Part model, mm, in its own coordinate system. A direction names the side the tool comes from. Coordinates: 2 decimals unless noted, no trailing zeros. Loops run counter-clockwise (first coordinate to the right, second up) from the corner with the lowest first, then second, coordinate; pieces in that order, holes last. Notation, with made-up numbers: (-38, 33) - (-13, 33) arc R28 ccw to (-13, 54) - close; hole circle Ø10 at (75, 25). An arc over 180 degrees is marked (long way). Use a Markdown table: item, result. Add a question column.
1. Drop flat-ended pins along their axis: pin 1 (2 mm diameter, centred on x = -4.5, y = 5, fed in from -Z); pin 2 (5 mm diameter, centred on x = -4, y = 5, fed in from +Z); pin 3 (1 mm diameter, centred on x = 5, y = 7, fed in from +Z). Give the stop position or say it passes through.
2. Band-saw the part on D-D, the plane x = -3.75. Give the cut face in (y, z).
3. Band-saw the part on B-B, the plane x = 0. Give the cut face in (y, z), plus the area to 3 significant figures.
4. 3-axis set-ups, long thin cutter, end or side, ignore diameter. For faces 4 (the flat face through (-2, 8.5, 2)), 5 (the flat face through (-6, 7.25, 2)): which of +Z, -Z, +X, -X, +Y, -Y reach the whole face in a straight line?
5. Band-saw the part on C-C, the plane y = 1. Give the cut face in (x, z).
6. Wall check: probe 1 along X at (y, z) = (2, 0); probe 2 along Y at (x, z) = (-3.25, 6.25); probe 3 along Z at (x, y) = (0.25, 7). Give the ranges that are in metal, low to high. Write a range as [from, to].
7. Band-saw the part on A-A, the plane z = 0. Give the cut face in (x, y).
8. Pull direction X, two halves, no side cores. Call faces 1 (the cylindrical face through (-2, 4, 0)), 2 (the flat face through (-2, 0, 2)), 3 (the cylindrical face through (2.703, 7.866, 8.584)): pulls with the +X half, pulls with the -X half, needs draft (parallel to the pull), parting line crosses it, or undercut.
from build123d import *

# Parameters (mm, degrees)
SKETCH1_R           = 9
BOSS_EXTRUDE1_DEPTH = 1.25
SKETCH2_R           = 6
BOSS_EXTRUDE2_DEPTH = 6
SKETCH3_R           = 9
BOSS_EXTRUDE3_DEPTH = 1.25
SKETCH4_R           = 2
CUT_EXTRUDE1_DEPTH  = 10.25


with BuildPart() as part:
    # Sketch1 → Boss-Extrude1 (new body)
    with BuildSketch(Plane(origin=(0, 0, 0), x_dir=(1, 0, 0), z_dir=(0, 1, 0))):
        with Locations(Location((0, 0, 0), (0, 0, 270))):
            Circle(SKETCH1_R)
    extrude(amount=BOSS_EXTRUDE1_DEPTH)

    # Sketch2 → Boss-Extrude2 (add)
    with BuildSketch(Plane(origin=(0, 1.25, 0), x_dir=(1, 0, 0), z_dir=(0, 1, 0))):
        with Locations(Location((0, 0, 0), (0, 0, 270))):
            Circle(SKETCH2_R)
    extrude(amount=BOSS_EXTRUDE2_DEPTH)

    # Sketch3 → Boss-Extrude3 (add)
    with BuildSketch(Plane(origin=(0, 7.25, 0), x_dir=(1, 0, 0), z_dir=(0, 1, 0))):
        with Locations(Location((0, 0, 0), (0, 0, 270))):
            Circle(SKETCH3_R)
    extrude(amount=BOSS_EXTRUDE3_DEPTH)

    # Sketch4 → Cut-Extrude1 (cut)
    with BuildSketch(Plane(origin=(0, 8.5, 0), x_dir=(1, 0, 0), z_dir=(0, 1, 0))):
        with Locations(Location((0, 0, 0), (0, 0, 270))):
            Circle(SKETCH4_R)
    extrude(amount=-CUT_EXTRUDE1_DEPTH, mode=Mode.SUBTRACT)


solid = part.part
Geometry check:
| question | item | result |
|---|---|---|
| 1 | pin 1 | stops at z = -4.87 |
| 1 | pin 2 | stops at z = 8.52 |
| 1 | pin 3 | stops at z = 7.76 |
| 2 | outline | (0, -8.18) - (1.25, -8.18) - (1.25, -4.68) - (7.25, -4.68) - (7.25, -8.18) - (8.5, -8.18) - (8.5, 8.18) - (7.25, 8.18) - (7.25, 4.68) - (1.25, 4.68) - (1.25, 8.18) - (0, 8.18) - close |
| 3 | outline | (0, -9) - (1.25, -9) - (1.25, -6) - (7.25, -6) - (7.25, -9) - (8.5, -9) - (8.5, -2) - (0, -2) - close; (0, 2) - (8.5, 2) - (8.5, 9) - (7.25, 9) - (7.25, 6) - (1.25, 6) - (1.25, 9) - (0, 9) - close |
| 3 | area | 83.0 mm^2 |
| 4 | face 4 | +Z, -Z, +X, -X, +Y |
| 4 | face 5 | none |
| 5 | outline | circle Ø18 at (0, 0); hole circle Ø4 at (0, 0) |
| 6 | probe 1 | x = [-6, -2], [2, 6] |
| 6 | probe 2 | y = [0, 1.25], [7.25, 8.5] |
| 6 | probe 3 | z = [-5.99, -1.98], [1.98, 5.99] |
| 7 | outline | (-9, 0) - (-2, 0) - (-2, 8.5) - (-9, 8.5) - (-9, 7.25) - (-6, 7.25) - (-6, 1.25) - (-9, 1.25) - close; (2, 0) - (9, 0) - (9, 1.25) - (6, 1.25) - (6, 7.25) - (9, 7.25) - (9, 8.5) - (2, 8.5) - close |
| 8 | face 1 | undercut |
| 8 | face 2 | needs draft |
| 8 | face 3 | parting line crosses it |
